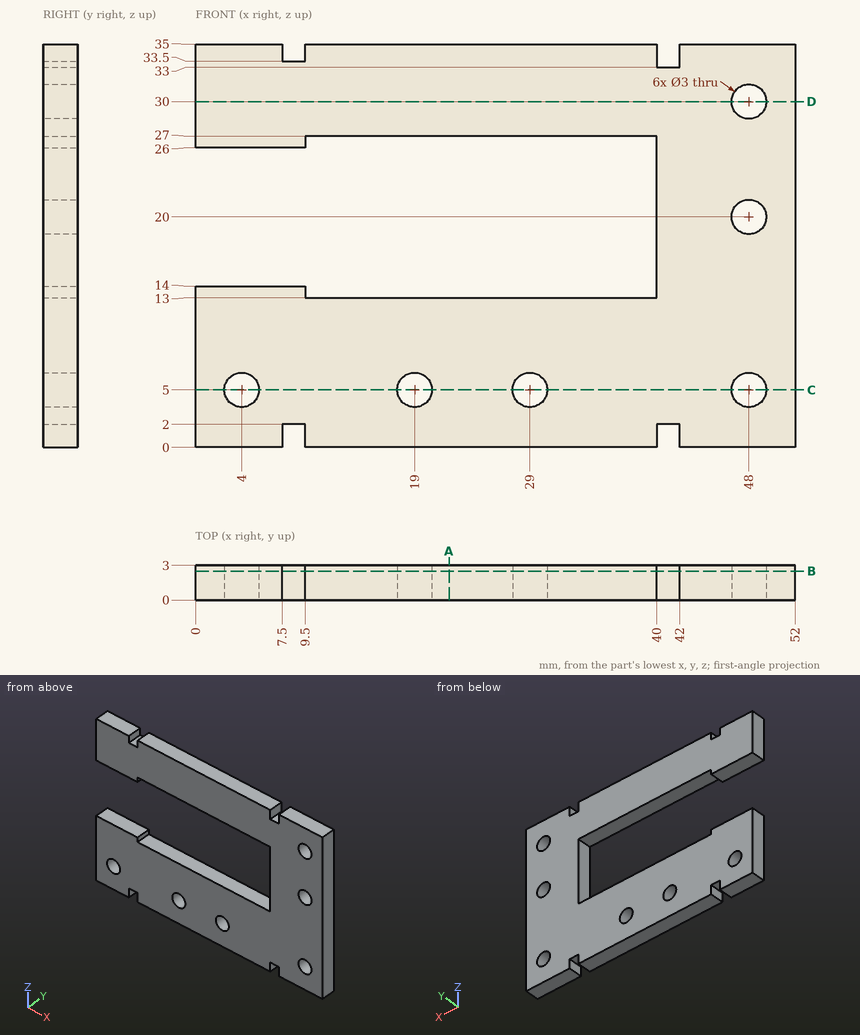
Design review of the part shown in the three views and the two pictorial views. Dimensions are in mm from the part's minimum x, y and z. Coordinates: 2 decimals unless noted, no trailing zeros. Write each loop counter-clockwise with the first axis right and the second up, starting at its lowest first coordinate (ties: lowest second). Pieces come first, ordered by that corner, then holes.
(1) Wall thickness on probe 1 along X at (y, z) = (1.7, 5); probe 2 along X at (y, z) = (1.6, 13.5); probe 3 along X at (y, z) = (2.4, 20): over which ranges is each line inside the solid? List them lowest first.
(2) Add section D-D on z = 30. Give the boundary of the cut face in (x, y), then the cut area to 3 significant figures.
(3) For pin 1 Ø1 at (y, z) = (2.5, 21.5) entering from -X; pin 2 Ø1.6 at (x, y) = (41, 1.5) entering from +Z; pin 3 Ø3.5 at (x, z) = (4, 5) entering from -Y, all flat-tipped, find the tip position at first contact; note any pin that passes through.
(4) Add section B-B on y = 2.5. Count the separate pieces of the cut face and the enclosed holes in it, then the cut area to 3 significant figures.
(5) Add section A-A on x = 22. Give the boundary of the cut face in (y, z), then the cut area to 3 significant figures.
(6) Add section C-C on z = 5. Give the boundary of the cut face in (x, y).
Answer sheet:
1. probe 1: x = 0 to 2.5, 5.5 to 17.5, 20.5 to 27.5, 30.5 to 46.5, 49.5 to 52
1. probe 2: x = 0 to 9.5, 40 to 52
1. probe 3: x = 40 to 46.5, 49.5 to 52
2. outline: (0, 0) - (46.5, 0) - (46.5, 3) - (0, 3) - close; (49.5, 0) - (52, 0) - (52, 3) - (49.5, 3) - close
2. area: 147 mm2
3. pin 1: stops at x = 40
3. pin 2: stops at z = 33
3. pin 3: stops at y = 0
4. separate pieces: 1
4. enclosed holes: 6
4. area: 1,220 mm2
5. outline: (0, 0) - (3, 0) - (3, 13) - (0, 13) - close; (0, 27) - (3, 27) - (3, 35) - (0, 35) - close
5. area: 63.0 mm2
6. outline: (0, 0) - (2.5, 0) - (2.5, 3) - (0, 3) - close; (5.5, 0) - (17.5, 0) - (17.5, 3) - (5.5, 3) - close; (20.5, 0) - (27.5, 0) - (27.5, 3) - (20.5, 3) - close; (30.5, 0) - (46.5, 0) - (46.5, 3) - (30.5, 3) - close; (49.5, 0) - (52, 0) - (52, 3) - (49.5, 3) - close
